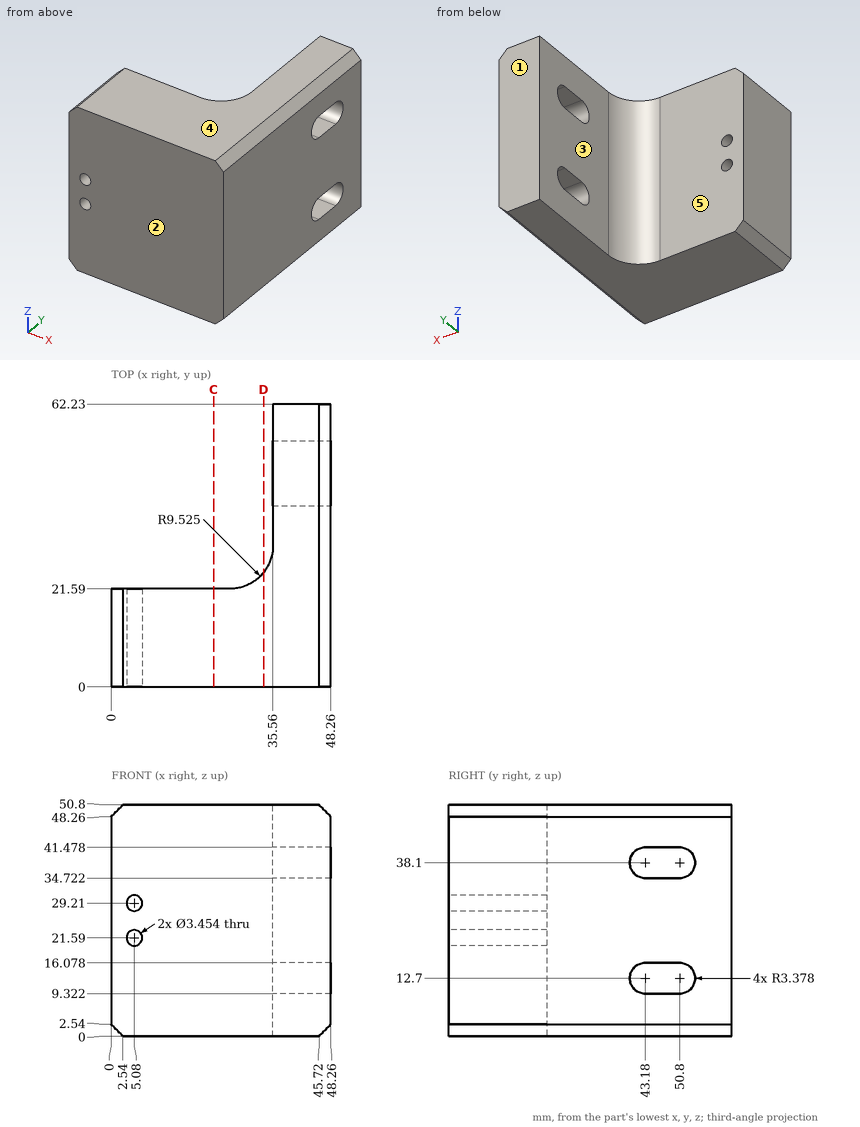
Drawing for the job (mm, zero at the part's lowest x, y, z). A direction names the side the tool comes from. Give positions to 0.01 mm unless a question says otherwise; leave off trailing zeros. Order: outer loops, then holes, each group sorted by start corner. A loop starts at its lowest first (then second) coordinate and runs counter-clockwise, first axis right, second up. Notation, with made-up numbers: (-16, -17) -> (4, -17) arc R26 ccw to (4, 12) -> close; hole circle Ø4 at (22.25, -40). An arc over 180 degrees is marked (long way). Use one line per item in the form item = value.
(1) Saw through at D-D (x = 33.5). Write the cut outline in (y, z).
Solution:
outline = (0, 0) -> (25.2, 0) -> (25.2, 50.8) -> (0, 50.8) -> close
(2) Pull direction Y, two halves, no side cores. Call the marked faces 1, 2 and 3: +Y half, -Y half, draft (parallel to the pull), parting line (faces both ways), or undercut.
Solution:
face_1 = +Y half
face_2 = -Y half
face_3 = draft
(3) Tool access for the marked faces 4 and 5: list every direction of +Z, -Z, +X, -X, +Y, -Y with a clear straight run to the whole face (end or side of a thin tool).
Solution:
face_4 = +Z, +X, -X, +Y, -Y
face_5 = +Z, -Z, -X, +Y
(4) Drill centre lines: line 1 (Z direction, x = 5.08, y = 8.5); line 2 (X direction, y = 15, z = 29) (1 decimal); line 3 (Z direction, x = 40.5, y = 49). Where is each one in solid material? Low to high. Write a range as from..to.
Solution:
line_1 = 0..19.86, 23.32..27.48, 30.94..50.8
line_2 = 0..3.4, 6.8..48.3
line_3 = 0..9.32, 16.08..34.72, 41.48..50.8
(5) Saw through at C-C (x = 22.5). Write the cut outline in (y, z).
Solution:
outline = (0, 0) -> (21.59, 0) -> (21.59, 50.8) -> (0, 50.8) -> close
(6) Flat gauge pins, fed straight in: P1, Ø6, axis at y = 27, z = 40, coming from the -X side; P2, Ø1.5, axis at x = 37.5, z = 40, coming from the -Y side; P3, Ø5.5, axis at x = 5.08, z = 29.21, coming from the +Y side; P4, Ø25, axis at y = 54, z = 37.5, coming from the -X side. Where does each tip first touch, or does it go through?
Solution:
P1 = 32.37
P2 = 0
P3 = 21.59
P4 = 35.56
